The model under review builds one solid part; all positions refer to its coordinate system, in mm. A direction names the side the tool comes from. Coordinates: 2 decimals unless noted, no trailing zeros. Write each loop counter-clockwise with the first axis right and the second up, starting at its lowest first coordinate (ties: lowest second). Pieces come first, ordered by that corner, then holes. Notation, with made-up numbers: M -3,5.5 L 45,5.5 A25 cw 45,28.5 Z; hole C -22,21.25 d1. An arc over 180 degrees is marked long. Answer as CSV lines item,"result". Start each with the question number.
from build123d import *

# Parameters (mm, degrees)
RESSALTO_EXTRUS_O1_DEPTH = 4
M3_CLEARANCE_HOLE2_D     = 3.2
ESBO_O7_R                = 8.4
CORTE_EXTRUS_O1_DEPTH    = 10
M3_CLEARANCE_HOLE1_D     = 3.2
M3_CLEARANCE_HOLE3_D     = 3.2
FILETE1_R                = 5
M3_CLEARANCE_HOLE5_D     = 3.2
FILETE2_R                = 2
ESBO_O16_W               = 17.35833251
ESBO_O16_H               = 3.95
ESBO_O16_W_2             = 17.358332509
CUT_EXTRUDE1_DEPTH       = 4
FILLET2_R                = 5


with BuildPart() as part:
    # Esboço1 → Ressalto-extrusão1 (new body)
    with BuildSketch(Plane.XY):
        with BuildLine():
            Line((-95.048931647, 26.894793301), (-95.048931647, 18.252242094))
            Line((-95.048931647, 18.252242094), (-115.048931647, 18.252242094))
            Line((-115.048931647, 18.252242094), (-115.048931647, 26.894793301))
            ThreePointArc((-115.048931647, 26.894793301), (-116.548931647, 30.0172923), (-115.048931647, 33.139791299))
            Line((-115.048931647, 33.139791299), (-115.048931647, 42.894793301))
            ThreePointArc((-115.048931647, 42.894793301), (-116.548931647, 46.0172923), (-115.048931647, 49.139791299))
            Line((-115.048931647, 49.139791299), (-115.048931647, 84.40808297))
            Line((-115.048931647, 84.40808297), (113.954781763, 84.40808297))
            Line((113.954781763, 84.40808297), (113.954781763, 49.139791299))
            ThreePointArc((113.954781763, 49.139791299), (115.454781763, 46.0172923), (113.954781763, 42.894793301))
            Line((113.954781763, 42.894793301), (113.954781763, 33.139791299))
            ThreePointArc((113.954781763, 33.139791299), (115.454781763, 30.0172923), (113.954781763, 26.894793301))
            Line((113.954781763, 26.894793301), (113.954781763, 18.252242094))
            Line((113.954781763, 18.252242094), (93.954781763, 18.252242094))
            Line((93.954781763, 18.252242094), (93.954781763, 26.894793301))
            ThreePointArc((93.954781763, 26.894793301), (92.454781763, 30.0172923), (93.954781763, 33.139791299))
            Line((93.954781763, 33.139791299), (93.954781763, 41.612292304))
            Line((93.954781763, 41.612292304), (73.826556743, 41.612292304))
            Line((73.826556743, 41.612292304), (70.826556743, 44.612292304))
            Line((70.826556743, 44.612292304), (70.826556743, 57.286376167))
            Line((70.826556743, 57.286376167), (-93.548931647, 56.342842726))
            Line((-93.548931647, 56.342842726), (-93.548931647, 46.0172923))
            ThreePointArc((-93.548931647, 46.0172923), (-93.999283778, 44.173383409), (-95.248931647, 42.744678666))
            Line((-95.248931647, 42.744678666), (-95.248931647, 33.289905934))
            ThreePointArc((-95.248931647, 33.289905934), (-93.550886325, 30.142326699), (-95.048931647, 26.894793301))
        make_face()
    extrude(amount=RESSALTO_EXTRUS_O1_DEPTH)

    # M3 Clearance Hole2 (through all)
    with Locations(Plane.XY.offset(4)):
        with Locations((-112.548931647, 46.0172923), (-112.548931647, 30.0172923), (-97.548931647, 30.0172923), (-97.548931647, 46.0172923), (96.454781763, 30.0172923), (111.454781763, 30.0172923), (111.454781763, 46.06544156), (96.454781763, 46.0172923)):
            Hole(M3_CLEARANCE_HOLE2_D / 2)

    # Esboço7 → Corte-extrusão1 (cut)
    with BuildSketch(Plane(origin=(0, 0, 0), x_dir=(-1, 0, 0), z_dir=(0, 0, -1))):
        with Locations((-91.876556743, 62.662292304)):
            Circle(ESBO_O7_R)
    extrude(amount=-CORTE_EXTRUS_O1_DEPTH, mode=Mode.SUBTRACT)

    # M3 Clearance Hole1 (through all)
    with Locations(Plane(origin=(0, 0, 0), x_dir=(-1, 0, 0), z_dir=(0, 0, -1))):
        with Locations((98.016827352, 62.117292304)):
            Hole(M3_CLEARANCE_HOLE1_D / 2)

    # M3 Clearance Hole3 (through all)
    with Locations(Plane(origin=(0, 0, 0), x_dir=(-1, 0, 0), z_dir=(0, 0, -1))):
        with Locations((-76.376556743, 47.162292304), (-76.376556743, 78.162292304), (-107.376556743, 78.162292304)):
            Hole(M3_CLEARANCE_HOLE3_D / 2)

    # Filete1
    filete1_edges = [part.edges().sort_by_distance(p)[0] for p in [
        (113.954781763, 33.139791299, 2),
        (113.954781763, 26.894793301, 2),
        (93.954781763, 26.894793301, 2),
        (93.954781763, 33.139791299, 2),
        (93.954781763, 41.612292304, 2),
        (70.826556743, 57.286376167, 2),
        (-95.248931647, 42.744678666, 2),
        (-95.248931647, 33.289905934, 2),
        (-95.048931647, 26.894793301, 2),
        (-115.048931647, 26.894793301, 2),
        (-115.048931647, 33.139791299, 2),
        (-115.048931647, 42.894793301, 2),
        (-115.048931647, 49.139791299, 2),
        (-115.048931647, 84.40808297, 2),
        (113.954781763, 84.40808297, 2),
        (113.954781763, 49.139791299, 2),
        (113.954781763, 42.894793301, 2),
    ]]
    fillet(filete1_edges, radius=FILETE1_R)

    # M3 Clearance Hole5 (through all)
    with Locations(Plane.XY.offset(4)):
        with Locations((-95.783895796, 79.917292304), (64.216104204, 79.917292304), (-15.783895796, 79.917292304)):
            Hole(M3_CLEARANCE_HOLE5_D / 2)

    # Filete2
    filete2_edges = [part.edges().sort_by_distance(p)[0] for p in [
        (113.954781763, 18.252242094, 2),
        (93.954781763, 18.252242094, 2),
        (73.826556743, 41.612292304, 2),
        (70.826556743, 44.612292304, 2),
        (-95.048931647, 18.252242094, 2),
        (-115.048931647, 18.252242094, 2),
    ]]
    fillet(filete2_edges, radius=FILETE2_R)

    # Esboço16 → Cut-Extrude1 (cut)
    with BuildSketch(Plane.XY.offset(4)):
        with Locations((-104.531590398, 22.092946092)):
            Rectangle(ESBO_O16_W, ESBO_O16_H)
        with Locations((103.437440514, 22.092946092)):
            Rectangle(ESBO_O16_W_2, ESBO_O16_H)
    extrude(amount=-CUT_EXTRUDE1_DEPTH, mode=Mode.SUBTRACT)

    # Fillet2
    fillet2_edges = [part.edges().sort_by_distance(p)[0] for p in [
        (-93.548931647, 56.342842726, 2),
    ]]
    fillet(fillet2_edges, radius=FILLET2_R)


solid = part.part
1) Clearance check with flat-ended pins moving along their axes: pin 1 Ø2 at (y, z) = (22.5, 2) entering from +X; pin 2 Ø0.8 at (y, z) = (36, 2) entering from -X. State where each tip first meets the part, or that it passes through.
2) Mouldability with a two-part tool opening along X and no side actions: class faces 4 (the flat face through (-115.049, 65, 2)), 5 (the cylindrical face through (92.45, 40.19, 2.03)), 6 (the flat face through (-2, 84.408, 2)) as +X half, -X half, draft (parallel to the pull), parting line (faces both ways), or undercut.
3) To check wall thickness, follow line 1 (X direction, y = 23, z = 3.35); line 2 (X direction, y = 33.5, z = 1.5); line 3 (X direction, y = 33, z = 3.45). State the ranges of each line that lie inside material, in increasing order. Write a range as [from, to].
4) Take a section at C-C on x = 28.5. Give the boundary of the cut face in (y, z), and give its area (3 significant figures).
5) Take a section at A-A on y = 68. Give the boundary of the cut face in (x, z).
6) Take a section at B-B on z = 0.9. Give the number of separate pieces and of enclosed holes in the cut face, and give its area (3 significant figures).
7) Take a section at D-D on x = -1.5. Give the boundary of the cut face in (y, z), and give its area (3 significant figures).
8) Tool access review of faces 1 (the flat face through (-95.852, 22, 2)), 2 (the flat face through (82, 41.612, 2)), 3 (the flat face through (-115.049, 23, 2)): name each direction out of +Z, -Z, +X, -X, +Y, -Y from which nothing blocks a thin tool from reaching the whole face with its end or side.
Results:
1,pin 1,"stops at x = 113.95"
1,pin 2,"stops at x = -115.05"
2,face 4,"-X half"
2,face 5,"undercut"
2,face 6,"draft"
3,line 1,"x = [-115.05, -113.21], [-95.85, -95.05], [93.95, 94.76], [112.12, 113.95]"
3,line 2,"x = [-115.28, -94.92], [93.73, 114.18]"
3,line 3,"x = [-115.46, -94.7], [93.54, 114.37]"
4,outline,"M 57.04,0 L 84.41,0 L 84.41,4 L 57.04,4 Z"
4,area,"109 mm²"
5,outline,"M -115.05,0 L 85.39,0 L 85.39,4 L -115.05,4 Z; M 98.36,0 L 113.95,0 L 113.95,4 L 98.36,4 Z"
6,separate pieces,"1"
6,enclosed holes,"18"
6,area,"7,790 mm²"
7,outline,"M 56.87,0 L 84.41,0 L 84.41,4 L 56.87,4 Z"
7,area,"110 mm²"
8,face 1,"+Z, -Z"
8,face 2,"+Z, -Z, -Y"
8,face 3,"+Z, -Z, -X, -Y"
